Autodesk Inventor part; units mm, degrees
ref_plane "YZ Plane" through (0, 0, 0) normal (1, 0, 0) x (0, 1, 0)
ref_plane "XZ Plane" through (0, 0, 0) normal (0, 1, 0) x (-1, 0, 0)
ref_plane "XY Plane" through (0, 0, 0) normal (0, 0, 1) x (1, 0, 0)
ref_plane "Arbeitsebene1" through (0, 0, 0) normal (0, 0, 1) x (1, 0, 0)
sketch "Skizze1" plane through (0, 0, 0) normal (0, 0, 1) x (1, 0, 0)
  circle A0 centre (86.3298, 4) radius 1.4
  circle A1 centre (24.4799, 20.3) radius 1.4
  circle A2 centre (52.4799, 20.3) radius 1.4
  circle A3 centre (52.4799, 6.2) radius 1.4
  circle A4 centre (24.4799, 6.2) radius 1.4
  circle A5 centre (7.3298, 20.3) radius 1.4
  circle A6 centre (7.3298, 4) radius 1.4
  line L0 (90, 24.3) -> (90, 0)
  line L1 (89.0152, 24.3) -> (90, 24.3)
  line L2 (89.0152, 24.3) -> (89.0152, 10)
  line L3 (89.0152, 10) -> (59.35, 10)
  line L4 (59.35, 10) -> (59.35, 24.3)
  line L5 (5, 24.3) -> (59.35, 24.3)
  line L6 (5, 0) -> (5, 24.3)
  line L7 (5, 0) -> (90, 0)
  line L8 (6, 48.6) -> (6, 24.3)
  line L9 (6, 24.3) -> (60.35, 24.3)
  line L10 (60.35, 38.6) -> (60.35, 24.3)
  line L11 (89.95, 38.6) -> (60.35, 38.6)
  line L12 (89.95, 24.3) -> (89.95, 38.6)
  line L13 (89.95, 24.3) -> (91, 24.3)
  line L14 (91, 24.3) -> (91, 48.6)
  line L15 (6, 48.6) -> (91, 48.6)
  line L16 (21.4799, 24.3) -> (57.4799, 24.3)
  line L17 (57.4799, 24.3) -> (57.4799, 14.3)
  line L18 (57.4799, 14.3) -> (21.4799, 14.3)
  line L19 (21.4799, 14.3) -> (21.4799, 24.3)
  point P0 (0, 0)
  dimension "d0" = 36
  dimension "d1" = 10
  dimension "d2" = 3
extrude "Extrusion1" add sketch "Skizze1" along normal blind 5 contours L5 L17 L18 L19
fillet "Rundung1" radius 2 2 edges at (21.4799, 14.3, 2.5) (57.4799, 14.3, 2.5)
mirror "Spiegeln1" about plane through (57.4799, 24.3, 0) normal (0, 1, 0) of "Extrusion1", "Rundung1"
properties part number "60_Planktoscope_Cabletie"
Here's how the part is built. I have some questions about the finished solid (model axes, mm). Coordinates: 2 decimals unless noted, no trailing zeros. Loops run counter-clockwise (first coordinate to the right, second up) from the corner with the lowest first, then second, coordinate; pieces in that order, holes last. Notation, with made-up numbers: M 50.25,-14 L 101.25,-14 A14 ccw 101.25,4 Z; hole C 30,73.5 d7. An arc over 180 degrees is marked long. One line per item, written item: value.
1. Imagine slicing it at A-A (y = 20.3). List the corners of the cut face in (x, z) for me, and give its area (3 significant figures).
Geometry says:
outline: M 21.48,0 L 23.08,0 L 23.08,5 L 21.48,5 Z; M 25.88,0 L 51.08,0 L 51.08,5 L 25.88,5 Z; M 53.88,0 L 57.48,0 L 57.48,5 L 53.88,5 Z
area: 152 mm2
2. Will this pin go through, and if not, where does the flat tip stop? pin 1 Ø3.5 at (x, y) = (24.48, 20.3) entering from -Z.
Geometry says:
pin 1: stops at z = 0
3. Please list where these lines run through material, in increasing order: probe 1 along X at (y, z) = (28.3, 2.5); probe 2 along Y at (x, z) = (25.5, 1.35); probe 3 along X at (y, z) = (20, 1.6).
Geometry says:
probe 1: x = 21.48 to 23.08, 25.88 to 51.08, 53.88 to 57.48
probe 2: y = 14.3 to 19.34, 21.26 to 27.34, 29.26 to 34.3
probe 3: x = 21.48 to 23.11, 25.85 to 51.11, 53.85 to 57.48
4. Thinking about a two-plate mould opening in Y: for faces 1 (the cylindrical face through (56.91, 33.7, 2.54)), 2 (the cylindrical face through (51.08, 20.24, 2.46)), 3 (the cylindrical face through (23.45, 27.35, 2.46)), 4 (the flat face through (57.48, 24, 2)), which applies, +Y half, -Y half, draft (parallel to the pull), parting line (faces both ways), or undercut?
Geometry says:
face 1: +Y half
face 2: undercut
face 3: undercut
face 4: draft
5. Imagine slicing it at B-B (z = 1.85). List the corners of the cut face in (x, y) for me, and give its area (3 significant figures).
Geometry says:
outline: M 21.48,16.3 A2 ccw 23.48,14.3 L 55.48,14.3 A2 ccw 57.48,16.3 L 57.48,32.3 A2 ccw 55.48,34.3 L 23.48,34.3 A2 ccw 21.48,32.3 Z; hole C 24.48,20.3 d2.8; hole C 24.48,28.3 d2.8; hole C 52.48,20.3 d2.8; hole C 52.48,28.3 d2.8
area: 692 mm2
